Can you work these out from the model? Positions are in its coordinate system, mm. A direction names the side the tool comes from. Round coordinates to 2 decimals unless told otherwise and drop trailing zeros. Write each loop counter-clockwise with the first axis right and the second up, starting at its lowest first coordinate (ties: lowest second). Pieces come first, ordered by that corner, then holes.
Q1. If we section it at B-B (y = 0): Please give me the cut outline in (x, z) (3 decimals).
Q2. If we section it at A-A (z = 5.5): Please give me the cut outline in (x, y) (3 decimals), plus the area to 3 significant figures.
Q3. I'm going to push flat-ended pins straight in: pin 1 Ø6.5 at (x, y) = (-5, -23) entering from +Z; pin 2 Ø1.4 at (y, z) = (6.5, 6.5) entering from +X; pin 3 Ø2.5 at (x, z) = (-6.5, 1) entering from +Y; pin 4 Ø3.5 at (x, y) = (0, 0) entering from -Z. Where does each tip first touch, or does it pass through?
Q4. If we section it at D-D (z = 1.25): Please give me the cut outline in (x, y) (3 decimals).
Q5. If we section it at C-C (x = 0): Please give me the cut outline in (y, z) (3 decimals).
Q6. Please list where these lines run through material, in increasing order: line 1 along X through (y, z) = (0, 2.85) (3 decimals); line 2 along Y through (x, z) = (0, 1.7) (3 decimals).
Q7. For faces 1 (the flat face through (-4.1, -6, 6)), 2 (the flat face through (-6, -20.815, 1)), 3 (the flat face through (-7.2, -23, 1)), 4 (the flat face through (-12, 4.25, 6)), which set-ups out of +Z, -Z, +X, -X, +Y, -Y let a thin tool reach every point of the face, with its end or its side?
Q8. We'd pull the mould along X, two halves only. Please class faces 5 (the cylindrical face through (-0.596, 2.685, 1.824)), 6 (the flat face through (1.15, -23, 1)), 7 (the flat face through (4.1, 6, 6)), 8 (the flat face through (0, -10, 7.7)): +X half, -X half, draft (parallel to the pull), parting line (faces both ways), or undercut.
from build123d import *

# Parameters (mm, degrees)
F0_R     = 19.815
F1_DEPTH = 7.7
F2_W     = 8.2
F2_H     = 14
F3_DEPTH = 4
F4_W     = 40.63
F4_H     = 8.5
F5_DEPTH = 4
F6_W     = 2.3
F6_H     = 2.3
F6_W_2   = 3.75
F6_H_2   = 2.7
F7_DEPTH = 2.3
F8_R     = 2.75
F9_DEPTH = 25


with BuildPart() as f1:
    # F0 (on Top) → F1 (new body)
    with BuildSketch(Plane.XY):
        Circle(F0_R)
    extrude(amount=F1_DEPTH)

    # F2 (on face) → F3 (cut)
    with BuildSketch(Plane.XY.offset(7.7)):
        Rectangle(F2_W, F2_H)
    extrude(amount=-F3_DEPTH, mode=Mode.SUBTRACT)

    # F4 (on face) → F5 (cut)
    with BuildSketch(Plane.XY.offset(7.7)):
        Rectangle(F4_W, F4_H)
    extrude(amount=-F5_DEPTH, mode=Mode.SUBTRACT)

    # F6 (on face) → F7 (join)
    with BuildSketch(Plane(origin=(0, 0, 0), x_dir=(1, 0, 0), z_dir=(0, 0, -1))):
        with Locations((0, 24.665)):
            Rectangle(F6_W, F6_H)
        with Locations((-3.025, 24.665)):
            Rectangle(F6_W_2, F6_H)
        Polygon((1.15, 19.815), (1.15, 23.515), (-1.15, 23.515), (-1.15, 19.815), (-1.15, 19.516828), (1.172135, 19.553192), align=None)
        with Locations((-6.05, 24.665)):
            Rectangle(F6_W, F6_H)
        with Locations((-6.05, 22.165)):
            Rectangle(F6_W, F6_H_2)
    extrude(amount=-F7_DEPTH)

    # F8 (on face) → F9 (cut)
    with BuildSketch(Plane(origin=(0, 0, 0), x_dir=(1, 0, 0), z_dir=(0, 0, -1))):
        Circle(F8_R)
    extrude(amount=-F9_DEPTH, mode=Mode.SUBTRACT)


solid = f1.part
A:
1. outline: (-19.815, 0) - (-2.75, 0) - (-2.75, 3.7) - (-19.815, 3.7) - close; (2.75, 0) - (19.815, 0) - (19.815, 3.7) - (2.75, 3.7) - close
2. outline: (-19.354, -4.25) arc R19.815 ccw to (19.354, -4.25) - (4.1, -4.25) - (4.1, -7) - (-4.1, -7) - (-4.1, -4.25) - close; (-19.354, 4.25) - (-4.1, 4.25) - (-4.1, 7) - (4.1, 7) - (4.1, 4.25) - (19.354, 4.25) arc R19.815 ccw to start
2. area: 854 mm2
3. pin 1: stops at z = 2.3
3. pin 2: stops at x = 18.95
3. pin 3: stops at y = 19.11
3. pin 4: passes through
4. outline: (-7.2, -25.815) - (1.15, -25.815) - (1.15, -19.815) - (1.153, -19.781) arc R19.815 ccw (long way) to (-1.15, -19.782) - (-1.15, -23.515) - (-4.9, -23.515) - (-4.9, -20.815) - (-7.2, -20.815) - close; hole circle Ø5.5 at (0, 0)
5. outline: (-25.815, 0) - (-2.75, 0) - (-2.75, 3.7) - (-7, 3.7) - (-7, 7.7) - (-19.815, 7.7) - (-19.815, 2.3) - (-25.815, 2.3) - close; (2.75, 0) - (19.815, 0) - (19.815, 7.7) - (7, 7.7) - (7, 3.7) - (2.75, 3.7) - close
6. line 1: x = -19.815 to -2.75, 2.75 to 19.815
6. line 2: y = -25.815 to -2.75, 2.75 to 19.815
7. face 1: +Z
7. face 2: +Z, -Z, -X
7. face 3: +Z, -Z, -X, -Y
7. face 4: +Z, +X, -X
8. face 5: undercut
8. face 6: +X half
8. face 7: undercut
8. face 8: draft
